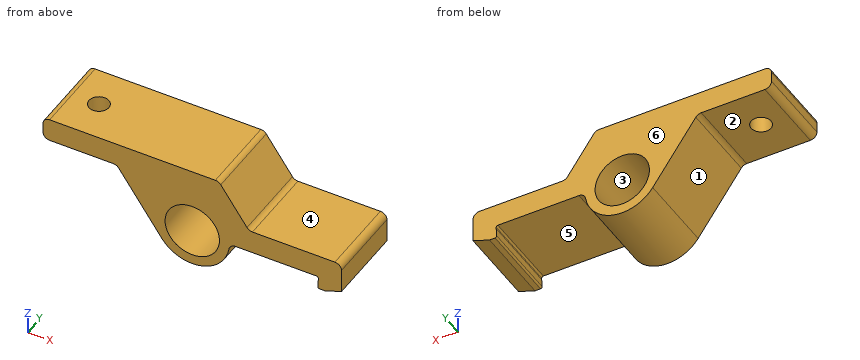
```python
from build123d import *

# Parameters (mm, degrees)
SKETCH1_R             = 4.1
BOSS_EXTRUDE1_DEPTH   = 6
F_3_0MM_DOWEL_HOLE1_D = 3
BOSS_EXTRUDE3_DEPTH   = 12
FILLET1_R             = 0.25
FILLET3_R             = 1
CUT_EXTRUDE3_DEPTH    = 12


with BuildPart() as part:
    # Sketch1 → Boss-Extrude1 (new, symmetric)
    with BuildSketch(Plane(origin=(0, 0, 0), x_dir=(1, 0, 0), z_dir=(0, 1, 0))):
        with BuildLine():
            Line((0, 0), (26.5, 0))
            Line((26.5, 0), (31.051348998, 6.5))
            Line((31.051348998, 6.5), (45, 6.5))
            Line((45, 6.5), (45, 12))
            Line((45, 12), (41.5, 12))
            Line((41.5, 12), (41.5, 10))
            Line((41.5, 10), (28.1, 10))
            ThreePointArc((28.1, 10), (24.183952477, 15.340814924), (17.912748552, 13.212028044))
            Line((17.912748552, 13.212028044), (11.112313305, 3.5))
            Line((11.112313305, 3.5), (0, 3.5))
            Line((0, 3.5), (0, 0))
        make_face()
        with Locations(Location((22.5, 10, 0), (0, 0, 270))):
            Circle(SKETCH1_R, mode=Mode.SUBTRACT)
    extrude(amount=BOSS_EXTRUDE1_DEPTH, both=True)

    # Ø3.0mm Dowel Hole1 (through all)
    with Locations(Plane.XY):
        with Locations((5, 0)):
            Hole(F_3_0MM_DOWEL_HOLE1_D / 2)

    # Sketch5 → Boss-Extrude3 (add)
    with BuildSketch(Plane(origin=(0, 6, 0), x_dir=(1, 0, 0), z_dir=(0, 1, 0))):
        with BuildLine():
            Line((41.5, 12), (41.5, 10.5))
            ThreePointArc((41.5, 10.5), (41.465364553, 11.250978566), (41.401058171, 12))
            Line((41.401058171, 12), (41.5, 12))
        make_face()
    extrude(amount=-BOSS_EXTRUDE3_DEPTH)

    # Fillet1
    fillet1_edges = [part.edges().sort_by_distance(p)[0] for p in [
        (41.5, 0, -10),
        (41.401058171, 0, -12),
    ]]
    fillet(fillet1_edges, radius=FILLET1_R)

    # Fillet3
    fillet3_edges = [part.edges().sort_by_distance(p)[0] for p in [
        (31.051348998, 0, -6.5),
        (26.5, 0, 0),
        (0, 0, 0),
        (0, 0, -3.5),
        (11.112313305, 0, -3.5),
        (28.1, 0, -10),
        (45, 0, -6.5),
    ]]
    fillet(fillet3_edges, radius=FILLET3_R)

    # Sketch8 → Cut-Extrude3 (cut)
    with BuildSketch(Plane(origin=(0, 6, 0), x_dir=(1, 0, 0), z_dir=(0, 1, 0))):
        Polygon((45, 12), (42.5, 12), (45, 11.090074414), align=None)
    extrude(amount=-CUT_EXTRUDE3_DEPTH, mode=Mode.SUBTRACT)


solid = part.part
```
Verification items for the finished model (mm, model axes). Face numbers are marked on the shaded views. A direction names the side the tool comes from. Coordinates: 2 decimals unless noted, no trailing zeros. Loops run counter-clockwise (first coordinate to the right, second up) from the corner with the lowest first, then second, coordinate; pieces in that order, holes last. Notation, with made-up numbers: (25.5, 14) -> (46.5, 14) arc R34 ccw to (46.5, 49) -> close; hole circle Ø10 at (56, 21.25). An arc over 180 degrees is marked (long way). Answer in a Markdown table with one row per item.
1) Draft check along X on the marked faces 1, 2 and 3. Enter one of: released by +X, released by -X, zero draft, split by the parting line, or undercut.
The answers:
| item | result |
|---|---|
| face 1 | released by -X |
| face 2 | zero draft |
| face 3 | undercut |
2) Section check D-D (x = 5). Record the cut outline in (y, z).
The answers:
| item | result |
|---|---|
| outline | (-6, -3.5) -> (-1.5, -3.5) -> (-1.5, 0) -> (-6, 0) -> close; (1.5, -3.5) -> (6, -3.5) -> (6, 0) -> (1.5, 0) -> close |
3) Scan lines: line 1 along Y through (x, z) = (5, -2.6); line 2 along X through (y, z) = (-1.25, -11); line 3 along Z through (x, y) = (31.5, 3.25). Record each from-to range of solid material in increasing order. Write a range as from..to.
The answers:
| item | result |
|---|---|
| line 1 | y = -6..-1.5, 1.5..6 |
| line 2 | x = 16.36..18.52, 26.48..28.01, 41.48..45 |
| line 3 | z = -10..-6.5 |
4) Access from +Z, -Z, +X, -X, +Y, -Y to the whole of each face (thin tool, end or side, straight path). Record for the marked faces 4, 5 and 6.
The answers:
| item | result |
|---|---|
| face 4 | +Z, +X, +Y, -Y |
| face 5 | -Z, +Y, -Y |
| face 6 | +Z, -Z, +X, -X, +Y |
5) Depth check by flat-ended pin: P1, Ø1.5, axis at x = 38, y = 2.5, coming from the -Z side; P2, Ø6, axis at y = 2, z = -5, coming from the +X side; P3, Ø5, axis at x = 5, y = 0, coming from the -Z side; P4, Ø1.5, axis at x = 36.5, y = -1, coming from the +Z side. Enter the tip coordinate at first touch or a pass-through.
The answers:
| item | result |
|---|---|
| P1 | stops at z = -10 |
| P2 | stops at x = 45 |
| P3 | stops at z = -3.5 |
| P4 | stops at z = -6.5 |
6) Section check A-A (y = 0). Record the cut outline in (x, z), and give its area (3 significant figures).
The answers:
| item | result |
|---|---|
| outline | (0, -2.5) arc R1 ccw to (1, -3.5) -> (3.5, -3.5) -> (3.5, 0) -> (1, 0) arc R1 ccw to (0, -1) -> close; (6.5, -3.5) -> (10.59, -3.5) arc R1 cw to (11.41, -3.93) -> (17.91, -13.21) arc R5.6 ccw to (28.04, -10.85) arc R1 cw to (29.02, -10) -> (41.25, -10) arc R0.25 cw to (41.5, -10.25) -> (41.5, -10.5) arc R19.01 cw to (41.43, -11.73) arc R0.25 ccw to (41.68, -12) -> (42.5, -12) -> (45, -11.09) -> (45, -7.5) arc R1 ccw to (44, -6.5) -> (31.57, -6.5) arc R1 cw to (30.75, -6.07) -> (26.8, -0.43) arc R1 ccw to (25.98, 0) -> (6.5, 0) -> close; hole circle Ø8.2 at (22.5, -10) |
| area | 250 mm2 |
7) Section check C-C (y = 2). Record the cut outline in (x, z).
The answers:
| item | result |
|---|---|
| outline | (0, -2.5) arc R1 ccw to (1, -3.5) -> (10.59, -3.5) arc R1 cw to (11.41, -3.93) -> (17.91, -13.21) arc R5.6 ccw to (28.04, -10.85) arc R1 cw to (29.02, -10) -> (41.25, -10) arc R0.25 cw to (41.5, -10.25) -> (41.5, -10.5) arc R19.01 cw to (41.43, -11.73) arc R0.25 ccw to (41.68, -12) -> (42.5, -12) -> (45, -11.09) -> (45, -7.5) arc R1 ccw to (44, -6.5) -> (31.57, -6.5) arc R1 cw to (30.75, -6.07) -> (26.8, -0.43) arc R1 ccw to (25.98, 0) -> (1, 0) arc R1 ccw to (0, -1) -> close; hole circle Ø8.2 at (22.5, -10) |
8) Section check B-B (x = 22.5). Record the cut outline in (y, z).
The answers:
| item | result |
|---|---|
| outline | (-6, -15.6) -> (6, -15.6) -> (6, -14.1) -> (-6, -14.1) -> close; (-6, -5.9) -> (6, -5.9) -> (6, 0) -> (-6, 0) -> close |
